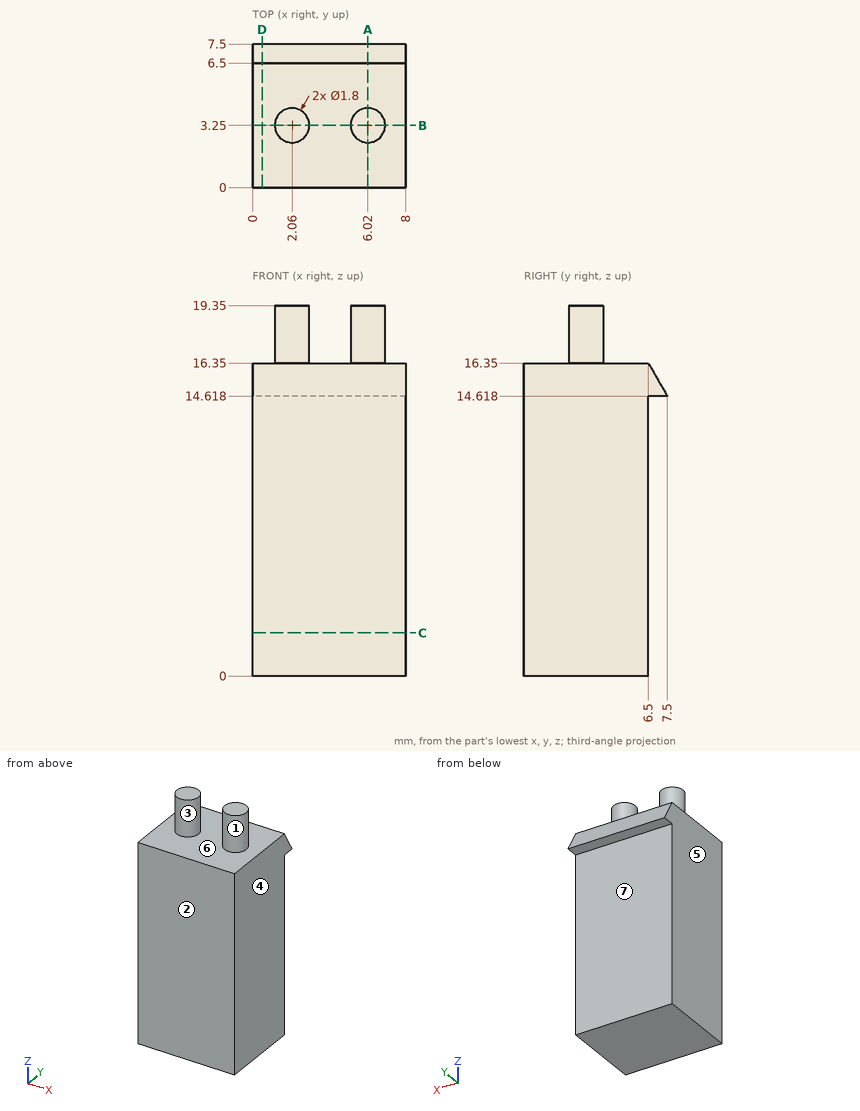
Verification items for this drawing (mm, ordinates from the low corner). A direction names the side the tool comes from. Give positions to 0.01 mm unless a question says otherwise; leave off trailing zeros. Loops run counter-clockwise (first coordinate to the right, second up) from the corner with the lowest first, then second, coordinate; pieces in that order, holes last. Notation, with made-up numbers: M -1,85.5 L 12,85.5 A18 ccw 12,120.5 Z; hole C 65.5,-39 d10. An arc over 180 degrees is marked long. Answer as a JSON object with one key per item and string values. Group by question number.
Item 1: Gauge pin test, flat end, axial feed: pin 1 (1.5 mm diameter, centred on x = 4, z = 10.5, fed in from +Y). Record the tip position at first contact, or that the pin passes through.
Item 2: Sectioned sample at B-B on y = 3.25. Record the boundary of the cut face in (x, z).
Item 3: Sectioned sample at A-A on x = 6.02. Record the boundary of the cut face in (y, z), plus the area to 3 significant figures.
Item 4: Sectioned sample at C-C on z = 2.25. Record the boundary of the cut face in (x, y), plus the area to 3 significant figures.
Item 5: Material ranges on L1, parallel to Z at x = 5, y = 0.5; L2, parallel to Y at x = 2.25, z = 4.25; L3, parallel to X at y = 3, z = 18, recorded low to high.
Item 6: Mould release check, pull along X, two halves, no side actions. Record for the marked faces 1, 2, 3 and 4: pulls with the +X half, pulls with the -X half, needs draft (parallel to the pull), parting line crosses it, or undercut.
Item 7: Access from +Z, -Z, +X, -X, +Y, -Y to the whole of each face (thin tool, end or side, straight path). Record for the marked faces 5, 6 and 7.
Item 8: Sectioned sample at D-D on x = 0.5. Record the boundary of the cut face in (y, z).
Findings below:
{
 "1": {"pin 1": "y = 6.5"},
 "2": {"outline": "M 0,0 L 8,0 L 8,16.35 L 6.92,16.35 L 6.92,19.35 L 5.12,19.35 L 5.12,16.35 L 2.96,16.35 L 2.96,19.35 L 1.16,19.35 L 1.16,16.35 L 0,16.35 Z"},
 "3": {"outline": "M 0,0 L 6.5,0 L 6.5,14.62 L 7.5,14.62 L 6.5,16.35 L 4.15,16.35 L 4.15,19.35 L 2.35,19.35 L 2.35,16.35 L 0,16.35 Z", "area": "113 mm2"},
 "4": {"outline": "M 0,0 L 8,0 L 8,6.5 L 0,6.5 Z", "area": "52.0 mm2"},
 "5": {"L1": "0 to 16.35", "L2": "0 to 6.5", "L3": "1.2 to 2.92, 5.16 to 6.88"},
 "6": {"face 1": "undercut", "face 2": "needs draft", "face 3": "undercut", "face 4": "pulls with the +X half"},
 "7": {"face 5": "+Z, -Z, -X, +Y, -Y", "face 6": "+Z", "face 7": "-Z, +X, -X, +Y"},
 "8": {"outline": "M 0,0 L 6.5,0 L 6.5,14.62 L 7.5,14.62 L 6.5,16.35 L 0,16.35 Z"}
}
